Could you check a few things on this model? Use its own coordinates, in mm. Face numbers are marked on the shaded views. A direction names the side the tool comes from. Coordinates: 2 decimals unless noted, no trailing zeros. Loops run counter-clockwise (first coordinate to the right, second up) from the corner with the lowest first, then second, coordinate; pieces in that order, holes last.
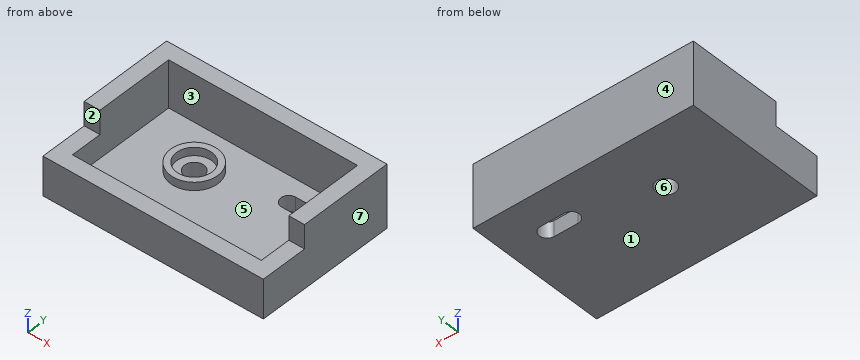
from build123d import *

# Parameters (mm, degrees)
F1_DEPTH = 25.4
F2_DEPTH = 15.748
F0_R     = 9.525
F3_DEPTH = 6.35
F0_R_2   = 7.112
F4_DEPTH = 9.652
F0_R_3   = 3.937
F5_DEPTH = 6.35


with BuildPart() as f1:
    # F0 (on Top) → F1 (new body)
    with BuildSketch(Plane.XY):
        Polygon((57.15, 23.622), (-31.75, 23.622), (-31.75, -14.478), (-25.4, -14.478), (-25.4, 17.272), (50.8, 17.272), (50.8, -14.478), (57.15, -14.478), align=None)
    extrude(amount=F1_DEPTH)

    # F0 (on Top) → F2 (join)
    with BuildSketch(Plane.XY):
        Polygon((-25.4, -14.478), (-31.75, -14.478), (-31.75, -33.528), (57.15, -33.528), (57.15, -14.478), (50.8, -14.478), (50.8, -27.178), (-25.4, -27.178), align=None)
    extrude(amount=F2_DEPTH)

    # F0 (on Top) → F3 (join)
    with BuildSketch(Plane.XY):
        Polygon((-25.4, 17.272), (-25.4, -14.478), (-25.4, -27.178), (50.8, -27.178), (50.8, -14.478), (50.8, 17.272), align=None)
        Circle(F0_R, mode=Mode.SUBTRACT)
        with BuildLine():
            ThreePointArc((31.496, 4.445), (28.321, 7.62), (31.496, 10.795))
            Line((31.496, 10.795), (41.148, 10.795))
            ThreePointArc((41.148, 10.795), (44.323, 7.62), (41.148, 4.445))
            Line((41.148, 4.445), (31.496, 4.445))
        make_face(mode=Mode.SUBTRACT)
    extrude(amount=F3_DEPTH)

    # F0 (on Top) → F4 (join)
    with BuildSketch(Plane.XY):
        Circle(F0_R)
        Circle(F0_R_2, mode=Mode.SUBTRACT)
    extrude(amount=F4_DEPTH)

    # F0 (on Top) → F5 (join)
    with BuildSketch(Plane.XY):
        Circle(F0_R_2)
        Circle(F0_R_3, mode=Mode.SUBTRACT)
    extrude(amount=F5_DEPTH)


solid = f1.part
1) Imagine slicing it at B-B on z = 3.5. List the corners of the cut face in (x, y) for me (3 decimals), plus the area to 3 significant figures.
2) Imagine slicing it at D-D on z = 20.75. List the corners of the cut face in (x, y) for me, plus the area to 3 significant figures.
3) If I drill on L1, parallel to Y at x = 0, z = 7.9 (3 decimals); L2, parallel to Y at x = 41.5, z = 5; L3, parallel to X at y = 11, z = 12.5, over which ranges is the centre line in solid material (lowest first)?
4) We'd pull the mould along X, two halves only. Please class the marked faces 4, 5, 6 and 7: released by +X, released by -X, zero draft, split by the parting line, or undercut.
5) Imagine slicing it at C-C on y = 0. List the corners of the cut face in (x, z) for me (3 decimals), plus the area to 3 significant figures.
6) Imagine slicing it at A-A on x = 0. List the corners of the cut face in (y, z) for me (3 decimals), plus the area to 3 significant figures.
7) For the marked faces 1, 2 and 3, which set-ups out of +Z, -Z, +X, -X, +Y, -Y let a thin tool reach every point of the face, with its end or its side?
8) Will these pins go through, and if not, where does the flat tip stop? pin 1 (3 mm diameter, centred on x = 5.5, y = -17, fed in from +Z); pin 2 (13.5 mm diameter, centred on x = 12.5, y = -9, fed in from +Z); pin 3 (1.9 mm diameter, centred on x = -28.5, z = 21.5, fed in from -Y).
Solved:
1. outline: (-31.75, -33.528) - (57.15, -33.528) - (57.15, 23.622) - (-31.75, 23.622) - close; hole circle Ø7.874 at (0, 0); hole (31.496, 4.445) - (41.148, 4.445) arc R3.175 ccw to (41.148, 10.795) - (31.496, 10.795) arc R3.175 ccw to start
1. area: 4,940 mm2
2. outline: (-31.75, -14.48) - (-25.4, -14.48) - (-25.4, 17.27) - (50.8, 17.27) - (50.8, -14.48) - (57.15, -14.48) - (57.15, 23.62) - (-31.75, 23.62) - close
2. area: 968 mm2
3. L1: y = -33.528 to -27.178, -9.525 to -7.112, 7.112 to 9.525, 17.272 to 23.622
3. L2: y = -33.53 to 4.46, 10.78 to 23.62
3. L3: x = -31.75 to -25.4, 50.8 to 57.15
4. face 4: zero draft
4. face 5: undercut
4. face 6: undercut
4. face 7: released by +X
5. outline: (-31.75, 0) - (-3.937, 0) - (-3.937, 6.35) - (-7.112, 6.35) - (-7.112, 9.652) - (-9.525, 9.652) - (-9.525, 6.35) - (-25.4, 6.35) - (-25.4, 25.4) - (-31.75, 25.4) - close; (3.937, 0) - (57.15, 0) - (57.15, 25.4) - (50.8, 25.4) - (50.8, 6.35) - (9.525, 6.35) - (9.525, 9.652) - (7.112, 9.652) - (7.112, 6.35) - (3.937, 6.35) - close
5. area: 772 mm2
6. outline: (-33.528, 0) - (-3.937, 0) - (-3.937, 6.35) - (-7.112, 6.35) - (-7.112, 9.652) - (-9.525, 9.652) - (-9.525, 6.35) - (-27.178, 6.35) - (-27.178, 15.748) - (-33.528, 15.748) - close; (3.937, 0) - (23.622, 0) - (23.622, 25.4) - (17.272, 25.4) - (17.272, 6.35) - (9.525, 6.35) - (9.525, 9.652) - (7.112, 9.652) - (7.112, 6.35) - (3.937, 6.35) - close
6. area: 509 mm2
7. face 1: -Z, +X, -X, +Y, -Y
7. face 2: +Z, +X, -X, -Y
7. face 3: +Z
8. pin 1: stops at z = 6.35
8. pin 2: stops at z = 9.65
8. pin 3: stops at y = -14.48
